Geometry: see drawing. Coordinates: mm, zero at the bounding-box minimum. A direction names the side the tool comes from. Round coordinates to 2 decimals unless told otherwise and drop trailing zeros. Write each loop counter-clockwise with the first axis right and the second up, starting at its lowest first coordinate (ties: lowest second). Pieces come first, ordered by that corner, then holes. Notation, with made-up numbers: (76.5, 61.5) -> (98.5, 61.5) arc R20 ccw to (98.5, 83.5) -> close; hole circle Ø4 at (47.25, 62). An arc over 180 degrees is marked (long way). Write item = value, one per line.
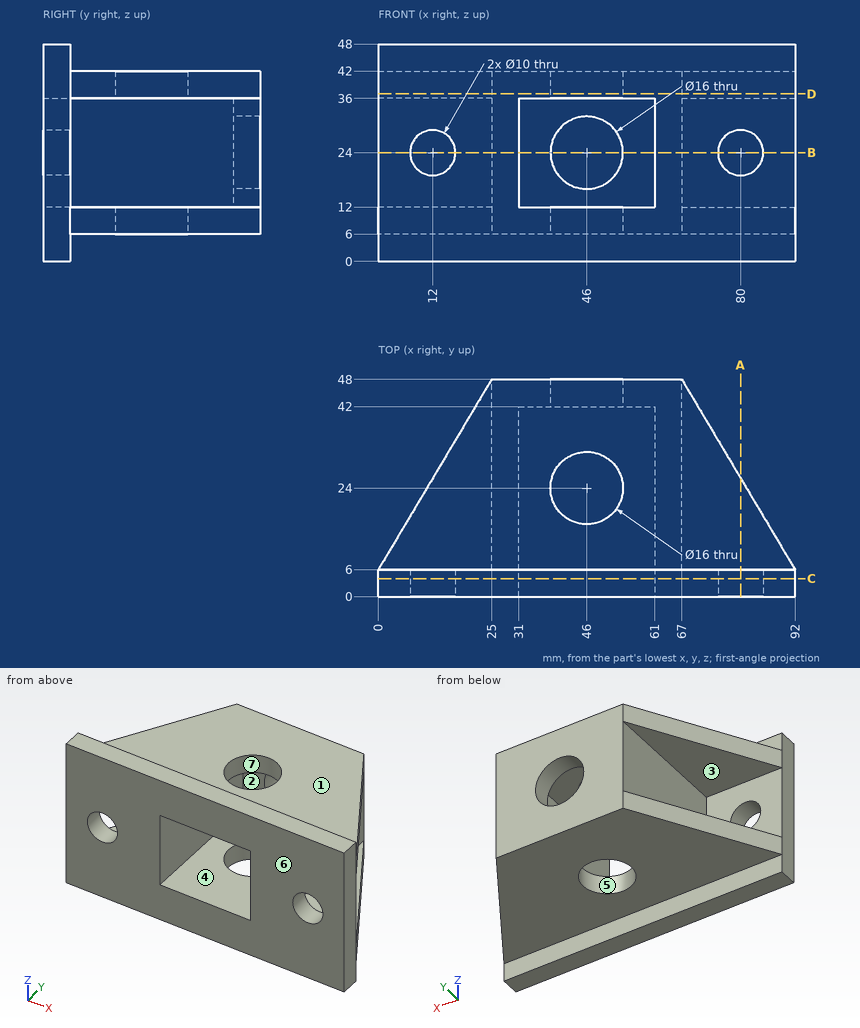
1) Cut plane D-D (z = 37). Return the cut outline in (x, y), and give its area (3 significant figures).
Solutions:
outline = (0, 0) -> (92, 0) -> (92, 6) -> (67, 48) -> (25, 48) -> (0, 6) -> close; hole circle Ø16 at (46, 24)
area = 3,160 mm^2
2) Cut plane B-B (z = 24). Return the cut outline in (x, y), and give its area (3 significant figures).
Solutions:
outline = (0, 0) -> (7, 0) -> (7, 6) -> (0, 6) -> close; (17, 0) -> (31, 0) -> (31, 42) -> (38, 42) -> (38, 48) -> (25, 48) -> (25, 6) -> (17, 6) -> close; (54, 42) -> (61, 42) -> (61, 0) -> (75, 0) -> (75, 6) -> (67, 6) -> (67, 48) -> (54, 48) -> close; (85, 0) -> (92, 0) -> (92, 6) -> (85, 6) -> close
area = 840 mm^2
3) Line query: L1, parallel to Z at x = 80, y = 3.15; L2, parallel to Z at x = 35.5, y = 17; L3, parallel to X at y = 38, z = 28. Output: solid intervals per line, ascending. Write a range as from..to.
Solutions:
L1 = 0..19, 29..48
L2 = 6..12, 36..42
L3 = 25..31, 61..67
4) Draft query along Y for the marked faces 4, 5, 6 and 7. Return one class per face: +Y half, -Y half, draft (parallel to the pull), parting line (faces both ways), or undercut.
Solutions:
face_4 = draft
face_5 = undercut
face_6 = -Y half
face_7 = undercut
5) First-contact query: P1, Ø12, axis at y = 31, z = 20, coming from the +X side; P2, Ø12.5, axis at x = 8, y = 27.5, coming from the -Z side; P3, Ø1.8, axis at x = 42, z = 4, coming from the +Y side. Flat tips, straight axial feed; report the tip coordinate or a pass-through.
Solutions:
P1 = 67
P2 = 6
P3 = 6
6) Cut plane C-C (y = 4). Return the cut outline in (x, z), and give its area (3 significant figures).
Solutions:
outline = (0, 0) -> (92, 0) -> (92, 48) -> (0, 48) -> close; hole circle Ø10 at (12, 24); hole (31, 12) -> (61, 12) -> (61, 36) -> (31, 36) -> close; hole circle Ø10 at (80, 24)
area = 3,540 mm^2
7) Access query for the marked faces 1, 2 and 3. Directions: +Z, -Z, +X, -X, +Y, -Y. A direction counts if a zero-diameter tool reaches every point of the face in a straight line with its end or side. Return the directions, or none.
Solutions:
face_1 = +Z, +X, -X, +Y
face_2 = -Y
face_3 = -X, +Y
8) Cut plane A-A (x = 80). Return the cut outline in (y, z).
Solutions:
outline = (0, 0) -> (6, 0) -> (6, 6) -> (26.16, 6) -> (26.16, 12) -> (6, 12) -> (6, 19) -> (0, 19) -> close; (0, 29) -> (6, 29) -> (6, 36) -> (26.16, 36) -> (26.16, 42) -> (6, 42) -> (6, 48) -> (0, 48) -> close
